Work out the finished part from the listing and answer in its coordinate system (mm). Give positions to 0.01 mm unless a question says otherwise; leave off trailing zeros. Loops run counter-clockwise (first coordinate to the right, second up) from the corner with the lowest first, then second, coordinate; pieces in that order, holes last. Notation, with made-up numbers: M 58.25,73.5 L 77.25,73.5 A27 ccw 77.25,111.5 Z; hole C 54,-14 d4. An arc over 180 degrees is marked long. Use a Markdown table: item, result.
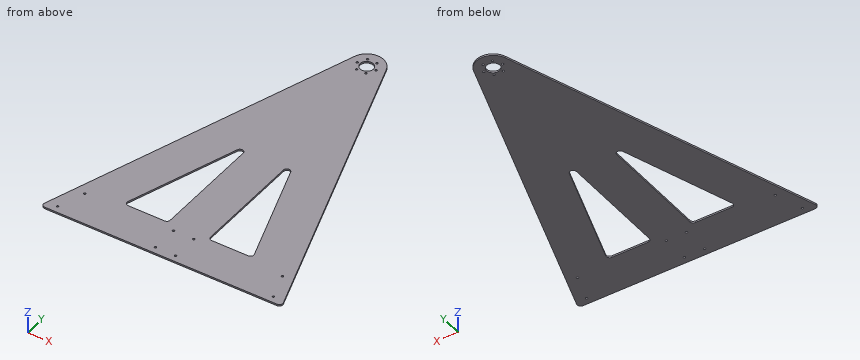
Autodesk Inventor part; units mm, degrees
ref_plane "YZ Plane" through (0, 0, 0) normal (1, 0, 0) x (0, 1, 0)
ref_plane "XZ Plane" through (0, 0, 0) normal (0, 1, 0) x (-1, 0, 0)
ref_plane "XY Plane" through (0, 0, 0) normal (0, 0, 1) x (1, 0, 0)
sketch "Sketch1" plane through (0, 0, 0) normal (0, 0, 1) x (1, 0, 0)
  circle A0 centre (-11, 0) radius 11
  circle A1 centre (-11, 0) radius 31.75
  line L0 (217.6, 31.75) -> (-239.6, 31.75)
  line L1 (-239.6, 31.75) -> (-239.6, -577.85)
  line L2 (-239.6, -577.85) -> (217.6, -577.85)
  line L3 (217.6, -577.85) -> (217.6, 31.75)
  line L4 (217.6, -577.85) -> (19.0819, 10.156)
  line L5 (-239.6, -577.85) -> (-41.0819, 10.156)
  line L6 (27.1, -501.65) -> (111.4484, -501.65)
  line L7 (111.4484, -501.65) -> (27.1, -251.8121)
  line L8 (27.1, -251.8121) -> (27.1, -501.65)
  line L9 (-11, 0) -> (-11, -6.454)
  line L10 (-49.1, -501.65) -> (-133.4484, -501.65)
  line L11 (-133.4484, -501.65) -> (-49.1, -251.8121)
  line L12 (-49.1, -251.8121) -> (-49.1, -501.65)
  circle A2 centre (193.2059, -565.15) radius 2
  circle A3 centre (176.0552, -514.35) radius 2
  circle A4 centre (8.05, -514.35) radius 2
  circle A5 centre (8.05, -565.15) radius 2
  circle A6 centre (-215.2059, -565.15) radius 2
  circle A7 centre (-198.0552, -514.35) radius 2
  circle A8 centre (-30.05, -514.35) radius 2
  circle A9 centre (-30.05, -565.15) radius 2
  circle A10 centre (-28.78, 0) radius 2
  circle A11 centre (-19.89, -15.3979) radius 2
  circle A12 centre (-2.11, -15.3979) radius 2
  circle A13 centre (6.78, 0) radius 2
  circle A14 centre (-2.11, 15.3979) radius 2
  circle A15 centre (-19.89, 15.3979) radius 2
  point P0 (0, 0)
  point P1 (-11, 31.75)
  point P2 (-11, -3.227)
  dimension "d0" = 63.5
  dimension "d1" = 457.2
  dimension "d2" = 609.6
  dimension "d3" = 76.2
  dimension "d4" = 76.2
  dimension "d5" = 38.1
  dimension "d6" = 4
  dimension "d7" = 4
  dimension "d8" = 4
  dimension "d9" = 4
  dimension "d10" = 12.7
  dimension "d11" = 12.7
  dimension "d12" = 19.05
  dimension "d13" = 19.05
  dimension "d14" = 19.05
  dimension "d15" = 4
  dimension "d16" = 17.78
  dimension "d19" = 360
extrude "Extrusion1" add sketch "Sketch1" against normal blind 3.175 contours A1 | A1 L4 L2 L5
fillet "Fillet1" radius 6.35 8 edges at (27.1, -251.8121, -1.5875) (-49.1, -251.8121, -1.5875) (111.4484, -501.65, -1.5875) (217.6, -577.85, -1.5875) (27.1, -501.65, -1.5875) (-49.1, -501.65, -1.5875) (-133.4484, -501.65, -1.5875) (-239.6, -577.85, -1.5875)
ref_plane "Work Plane1" through (-28.78, 0, -3.175) normal (0, 0.2588, -0.9659) x (1, 0, 0)
sketch "Sketch2" plane through (-28.78, 0, -3.175) normal (0, 0.2588, -0.9659) x (1, 0, 0)
  ellipse E0 centre (17.78, 0) end of major axis (6.7038, 0) minor radius 10.6988
  circle A0 centre (17.78, 0) radius 12.7
  dimension "d26" = 25.4
sketch "Sketch3" plane through (0, 0, -3.175) normal (0, 0, -1) x (-1, 0, 0)
  ellipse E0 centre (11, 0) end of major axis (-1.7, 0) minor radius 12.2673
  point P0 (0, 0)
extrude "Extrusion2" cut sketch "Sketch3" against normal through all
properties part number "FrameTop" material "MDF Medium Density Fiberboard"
(1) A cutting plane is placed at D-D (x = -154.5). Write down the section's boundary in (y, z) (3 decimals).
Entries:
| item | result |
|---|---|
| outline | M -577.85,-3.175 L -325.786,-3.175 L -325.786,0 L -577.85,0 Z |
(2) A cutting plane is placed at C-C (y = -52.5). Write down the section's boundary in (x, z) (3 decimals).
Entries:
| item | result |
|---|---|
| outline | M -62.235,-3.175 L 40.235,-3.175 L 40.235,0 L -62.235,0 Z |
(3) Given P1, Ø1.5, axis at y = -45.5, z = -2, coming from the +X side; P2, Ø1.5, axis at y = -99, z = -2, coming from the +X side, each flat-ended and moving along its own axis, determine where each tip first touches the part or whether it passes through.
Entries:
| item | result |
|---|---|
| P1 | stops at x = 38.13 |
| P2 | stops at x = 56.19 |
(4) Consider probe 1 along X at (y, z) = (-565.15, -1); probe 2 along X at (y, z) = (-408, -2.3); probe 3 along X at (y, z) = (-438, -1.45). Determine where each line is inside the solid, lowest interval first. Write a range as [from, to].
Entries:
| item | result |
|---|---|
| probe 1 | x = [-235.31, -217.21], [-213.21, -32.05], [-28.05, 6.05], [10.05, 191.21], [195.21, 213.31] |
| probe 2 | x = [-182.26, -101.83], [-49.1, 27.1], [79.83, 160.26] |
| probe 3 | x = [-192.38, -111.96], [-49.1, 27.1], [89.96, 170.38] |
(5) A cutting plane is placed at B-B (z = -0.6). Count the separate pieces of the cut face and the enclosed holes in it, and give its area (3 significant figures).
Entries:
| item | result |
|---|---|
| separate pieces | 1 |
| enclosed holes | 17 |
| area | 132,000 mm² |
(6) A cutting plane is placed at A-A (x = 77.5). Write down the section's boundary in (y, z) (3 decimals), and give its area (3 significant figures).
Entries:
| item | result |
|---|---|
| outline | M -577.85,-3.175 L -501.65,-3.175 L -501.65,0 L -577.85,0 Z; M -401.096,-3.175 L -162.877,-3.175 L -162.877,0 L -401.096,0 Z |
| area | 998 mm² |
